from build123d import *

# Parameters (mm, degrees)
F0_W     = 200
F0_H     = 50
F1_DEPTH = 25
F3_D     = 4
F4_D     = 6
F5_D     = 8
F6_D     = 10
F7_D     = 12
F8_D     = 16
F9_D     = 20


with BuildPart() as f1:
    # F0 (on Top) → F1 (new body, symmetric)
    with BuildSketch(Plane.XY):
        Rectangle(F0_W, F0_H)
    extrude(amount=F1_DEPTH, both=True)

    # F3 (through all)
    with Locations(Plane.XY.offset(25)):
        with Locations((-80, 0)):
            Hole(F3_D / 2)

    # F4 (through all)
    with Locations(Plane.XY.offset(25)):
        with Locations((-60, 0)):
            Hole(F4_D / 2)

    # F5 (through all)
    with Locations(Plane.XY.offset(25)):
        with Locations((-40, 0)):
            Hole(F5_D / 2)

    # F6 (through all)
    with Locations(Plane.XY.offset(25)):
        with Locations((-20, 0)):
            Hole(F6_D / 2)

    # F7 (through all)
    with Locations(Plane.XY.offset(25)):
        with Locations((0, 0)):
            Hole(F7_D / 2)

    # F8 (through all)
    with Locations(Plane.XY.offset(25)):
        with Locations((30, 0)):
            Hole(F8_D / 2)

    # F9 (through all)
    with Locations(Plane.XY.offset(25)):
        with Locations((60, 0)):
            Hole(F9_D / 2)


solid = f1.part
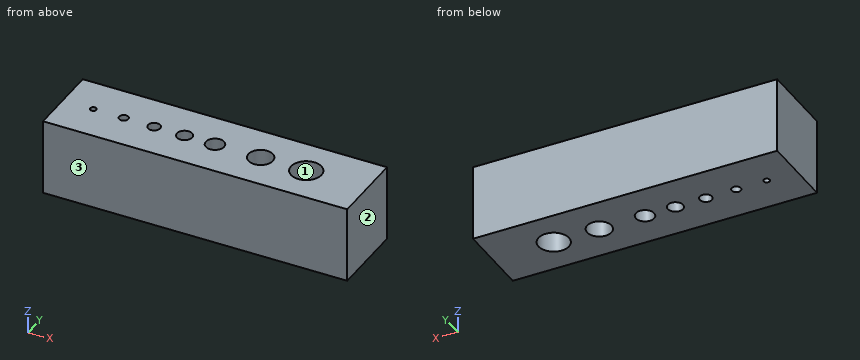
Design review of the part built by this model. Coordinates are the model's own, in mm. Face numbers are marked on the shaded views. Give positions to 0.01 mm unless a question says otherwise; leave off trailing zeros. Loops run counter-clockwise (first coordinate to the right, second up) from the corner with the lowest first, then second, coordinate; pieces in that order, holes last. Notation, with made-up numbers: (-38, 20.5) -> (-4, 20.5) arc R21 ccw to (-4, 39.5) -> close; hole circle Ø2 at (77.5, 65). An arc over 180 degrees is marked (long way). One line per question, with ' | ' between items. Start each with the question number.
(1) We need section D-D (x = -80). State the section outline as (y, z) points.
(2) We need section A-A (x = 0). State the section outline as (y, z) points, and give its area (3 significant figures).
(3) For line 1 (X direction, y = 5.5, z = 10); line 2 (Y direction, x = 30, z = 4); line 3 (Y direction, x = -20, z = -5.5), list the stretches that pass through material, from the lowest coordinate up.
(4) We need section B-B (y = 0). State how many separate pieces and enclosed holes the cut face has, and give its area (3 significant figures).
(5) We need section C-C (z = -19). State the section outline as (x, y) points, and give its area (3 significant figures).
(6) Draft analysis for pull direction X (two halves, no side actions). For the marked faces 1, 2 and 3, state which applies: +X half, -X half, draft (parallel to the pull), parting line (faces both ways), or undercut.
(7) Insertion check: P1, Ø6.5, axis at x = -40, y = 0, coming from the -Z side. The pin has a flat end and moves straight along its axis. Give the tip position at first contact, or say it passes through.
The answers:
1) outline: (-25, -25) -> (-2, -25) -> (-2, 25) -> (-25, 25) -> close; (2, -25) -> (25, -25) -> (25, 25) -> (2, 25) -> close
2) outline: (-25, -25) -> (-6, -25) -> (-6, 25) -> (-25, 25) -> close; (6, -25) -> (25, -25) -> (25, 25) -> (6, 25) -> close | area: 1,900 mm^2
3) line 1: x = -100 to -2.4, 2.4 to 24.19, 35.81 to 51.65, 68.35 to 100 | line 2: y = -25 to -8, 8 to 25 | line 3: y = -25 to -5, 5 to 25
4) separate pieces: 8 | enclosed holes: 0 | area: 6,200 mm^2
5) outline: (-100, -25) -> (100, -25) -> (100, 25) -> (-100, 25) -> close; hole circle Ø4 at (-80, 0); hole circle Ø6 at (-60, 0); hole circle Ø8 at (-40, 0); hole circle Ø10 at (-20, 0); hole circle Ø12 at (0, 0); hole circle Ø16 at (30, 0); hole circle Ø20 at (60, 0) | area: 9,200 mm^2
6) face 1: undercut | face 2: +X half | face 3: draft
7) P1: passes through
